Could you check a few things on this model? Use its own coordinates, in mm. A direction names the side the tool comes from. Coordinates: 2 decimals unless noted, no trailing zeros. Write each loop counter-clockwise with the first axis right and the second up, starting at its lowest first coordinate (ties: lowest second). Pieces come first, ordered by that corner, then holes.
```python
from build123d import *

# Parameters (mm, degrees)
SKETCH1_W           = 50
SKETCH1_H           = 16
BOSS_EXTRUDE1_DEPTH = 2
SKETCH2_R           = 2.325
BOSS_EXTRUDE2_DEPTH = 8
FILLET1_R           = 2
SKETCH3_W           = 20
SKETCH3_H           = 14
BOSS_EXTRUDE3_DEPTH = 3
SKETCH6_W           = 18
SKETCH6_H           = 2.7
CUT_EXTRUDE1_DEPTH  = 5


with BuildPart() as part:
    # Sketch1 → Boss-Extrude1 (new body)
    with BuildSketch(Plane.XY):
        with Locations((-5.32694175, 10.172569161)):
            Rectangle(SKETCH1_W, SKETCH1_H)
    extrude(amount=BOSS_EXTRUDE1_DEPTH)

    # Sketch2 → Boss-Extrude2 (add)
    with BuildSketch(Plane.XY.offset(2)):
        with Locations(Location((-24.675197488, 10.172569161, 0), (0, 0, 180))):
            Circle(SKETCH2_R)
        with Locations(Location((15.324802512, 10.172569161, 0), (0, 0, 180))):
            Circle(SKETCH2_R)
    extrude(amount=BOSS_EXTRUDE2_DEPTH)

    # Fillet1
    fillet1_edges = [part.edges().sort_by_distance(p)[0] for p in [
        (19.67305825, 2.172569161, 1),
        (-30.32694175, 2.172569161, 1),
        (-30.32694175, 18.172569161, 1),
        (19.67305825, 18.172569161, 1),
    ]]
    fillet(fillet1_edges, radius=FILLET1_R)

    # Sketch3 → Boss-Extrude3 (add)
    with BuildSketch(Plane(origin=(0, 0, 0), x_dir=(-1, 0, 0), z_dir=(0, 0, -1))):
        with Locations((5.32694175, 10.172569161)):
            Rectangle(SKETCH3_W, SKETCH3_H)
    extrude(amount=BOSS_EXTRUDE3_DEPTH)

    # Sketch6 → Cut-Extrude1 (cut)
    with BuildSketch(Plane(origin=(0, 0, -3), x_dir=(-1, 0, 0), z_dir=(0, 0, -1))):
        with Locations((5.32694175, 14.822569161)):
            Rectangle(SKETCH6_W, SKETCH6_H)
    extrude(amount=-CUT_EXTRUDE1_DEPTH, mode=Mode.SUBTRACT)


solid = part.part
```
1. On a 3-axis mill with a long thin cutter (end or side, diameter ignored), from which of +Z, -Z, +X, -X, +Y, -Y can I reach the whole of each face in a straight line? I mean faces 4 (the face through (-26.9, 9.5, 5.9)), 5 (the face through (4.673, 10, -1)), 6 (the face through (-5, 16.173, -1)). Say none if no direction works.
Verdict:
face 4: +Z
face 5: -Z, +X, +Y, -Y
face 6: +Z, -Z
2. I want a section at B-B on z = -1.5. Please give me the cut outline in (x, y), plus the area to 3 significant figures.
Verdict:
outline: (-15.33, 3.17) - (4.67, 3.17) - (4.67, 17.17) - (-15.33, 17.17) - close; hole (-14.33, 13.47) - (3.67, 13.47) - (3.67, 16.17) - (-14.33, 16.17) - close
area: 231 mm2
3. I want a section at D-D on z = 4. Please give me the cut outline in (x, y) (3 decimals), plus the area to 3 significant figures.
Verdict:
outline: circle Ø4.65 at (-24.675, 10.173); circle Ø4.65 at (15.325, 10.173)
area: 34.0 mm2
4. For pin 1 (1.4 mm diameter, centred on y = 15, z = -1.5, fed in from +X); pin 2 (1 mm diameter, centred on x = 13, y = 16, fed in from +Z); pin 3 (1.5 mm diameter, centred on x = -7, z = -1, fed in from -Y), each with a flat end and sliding along its axis, tell me the tip position at first contact or that it passes through.
Verdict:
pin 1: stops at x = 4.67
pin 2: stops at z = 2
pin 3: stops at y = 3.17
5. Please list where these lines run through material, in increasing order: line 1 along Y through (x, z) = (2.5, -1.5); line 2 along Z through (x, y) = (11, 8.75); line 3 along Z through (x, y) = (-13, 16.25).
Verdict:
line 1: y = 3.17 to 13.47, 16.17 to 17.17
line 2: z = 0 to 2
line 3: z = -3 to 2
6. I want a section at C-C on y = 5. Please give me the cut outline in (x, z).
Verdict:
outline: (-30.33, 0) - (-15.33, 0) - (-15.33, -3) - (4.67, -3) - (4.67, 0) - (19.67, 0) - (19.67, 2) - (-30.33, 2) - close
7. If we mould it in two halves opening along Y, with no side actions, what happens to faces 1 (the face through (-5, 13.473, -1)), 2 (the face through (-29.76, 17.57, 1.01)), 3 (the face through (19.673, 10, 1))? For each: pulls with the +Y half, pulls with the -Y half, needs draft (parallel to the pull), parting line crosses it, or undercut.
Verdict:
face 1: undercut
face 2: pulls with the +Y half
face 3: needs draft
8. I want a section at A-A on x = 2. Please give me the cut outline in (y, z).
Verdict:
outline: (2.17, 0) - (3.17, 0) - (3.17, -3) - (13.47, -3) - (13.47, 2) - (2.17, 2) - close; (16.17, -3) - (17.17, -3) - (17.17, 0) - (18.17, 0) - (18.17, 2) - (16.17, 2) - close
